The figure shows three views and two pictorial views of one solid part (mm, origin at its lowest corner). Answer the questions. Give positions to 0.01 mm unless a question says otherwise; leave off trailing zeros. Order: outer loops, then holes, each group sorted by start corner. A loop starts at its lowest first (then second) coordinate and runs counter-clockwise, first axis right, second up. Notation, with made-up numbers: (86, 47) - (93, 47) arc R24 ccw to (93, 68) - close; hole circle Ø10 at (-21.75, -20). An arc over 180 degrees is marked (long way). Answer as CSV lines item,"result". Start each with the question number.
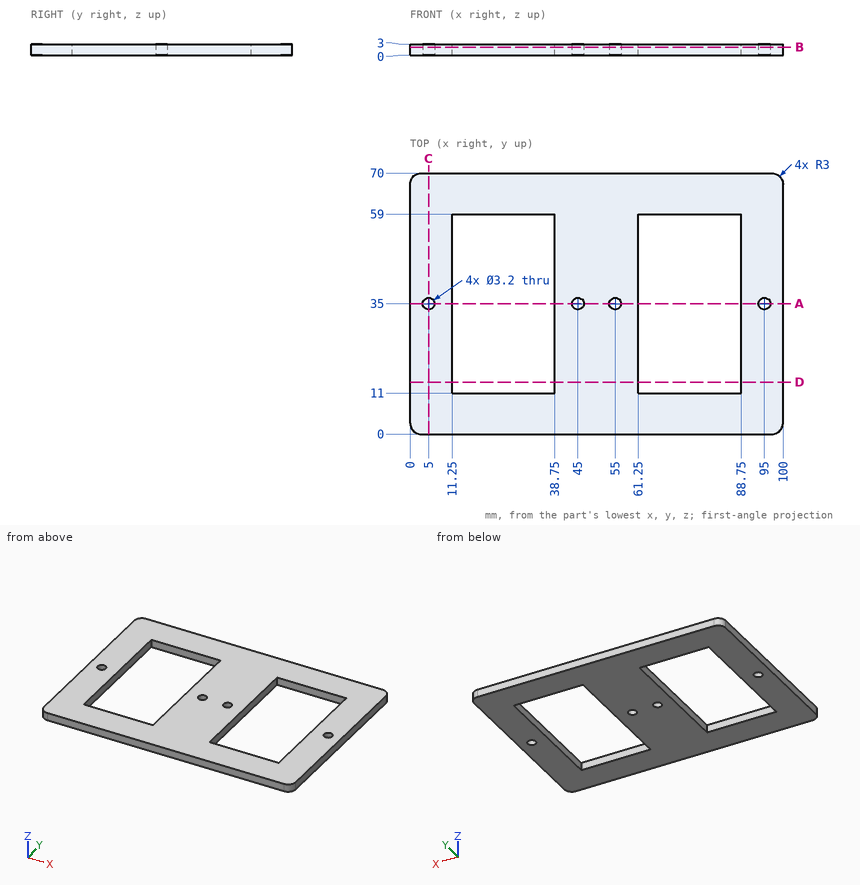
(1) Section C-C, the plane x = 5 is taken. Write down the section's boundary in (y, z), and give its area (3 significant figures).
(2) Section B-B, the plane z = 2.15 is taken. Write down the section's boundary in (x, y), and give its area (3 significant figures).
(3) Section D-D, the plane y = 14 is taken. Write down the section's boundary in (x, z), and give its area (3 significant figures).
(4) Section A-A, the plane y = 35 is taken. Write down the section's boundary in (x, z), and give its area (3 significant figures).
(5) Straight lines are drawn through the part: line 1 (X direction, y = 37.5, z = 1.4); line 2 (Y direction, x = 34, z = 2.4); line 3 (Y direction, x = 95, z = 2.05). For each, find the intervals that lie inside material, in ascending order. Write a range as [from, to].
Checks:
1,outline,"(0, 0) - (33.4, 0) - (33.4, 3) - (0, 3) - close; (36.6, 0) - (70, 0) - (70, 3) - (36.6, 3) - close"
1,area,"200 mm²"
2,outline,"(0, 3) arc R3 ccw to (3, 0) - (97, 0) arc R3 ccw to (100, 3) - (100, 67) arc R3 ccw to (97, 70) - (3, 70) arc R3 ccw to (0, 67) - close; hole circle Ø3.2 at (5, 35); hole (11.25, 11) - (38.75, 11) - (38.75, 59) - (11.25, 59) - close; hole circle Ø3.2 at (45, 35); hole circle Ø3.2 at (55, 35); hole (61.25, 11) - (88.75, 11) - (88.75, 59) - (61.25, 59) - close; hole circle Ø3.2 at (95, 35)"
2,area,"4,320 mm²"
3,outline,"(0, 0) - (11.25, 0) - (11.25, 3) - (0, 3) - close; (38.75, 0) - (61.25, 0) - (61.25, 3) - (38.75, 3) - close; (88.75, 0) - (100, 0) - (100, 3) - (88.75, 3) - close"
3,area,"135 mm²"
4,outline,"(0, 0) - (3.4, 0) - (3.4, 3) - (0, 3) - close; (6.6, 0) - (11.25, 0) - (11.25, 3) - (6.6, 3) - close; (38.75, 0) - (43.4, 0) - (43.4, 3) - (38.75, 3) - close; (46.6, 0) - (53.4, 0) - (53.4, 3) - (46.6, 3) - close; (56.6, 0) - (61.25, 0) - (61.25, 3) - (56.6, 3) - close; (88.75, 0) - (93.4, 0) - (93.4, 3) - (88.75, 3) - close; (96.6, 0) - (100, 0) - (100, 3) - (96.6, 3) - close"
4,area,"96.6 mm²"
5,line 1,"x = [0, 11.25], [38.75, 61.25], [88.75, 100]"
5,line 2,"y = [0, 11], [59, 70]"
5,line 3,"y = [0, 33.4], [36.6, 70]"
